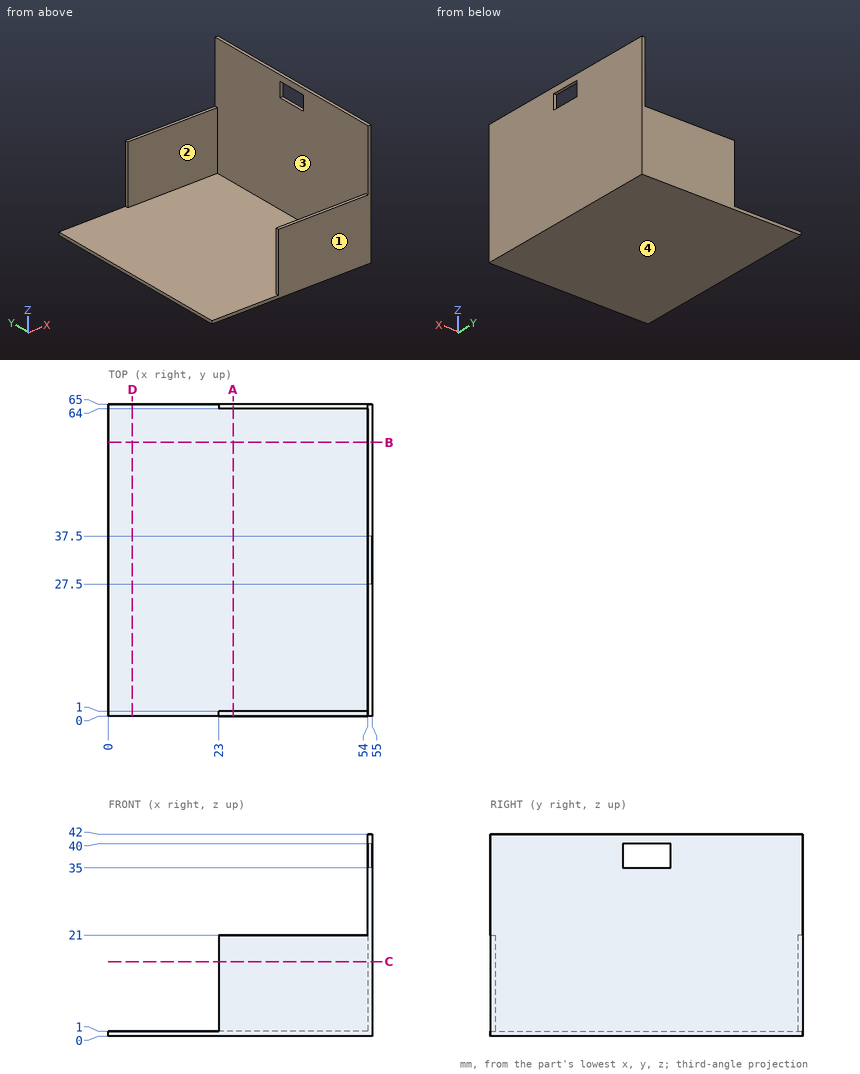
The drawing under review shows one solid part. Ordinate dimensions are in mm from its lowest x, y, z. Coordinates: 2 decimals unless noted, no trailing zeros. Write each loop counter-clockwise with the first axis right and the second up, starting at its lowest first coordinate (ties: lowest second). Pieces come first, ordered by that corner, then holes. Notation, with made-up numbers: (89, 38) -> (120, 38) arc R23 cw to (120, 47) -> close; hole circle Ø10 at (-24.75, 53). An arc over 180 degrees is marked (long way). One line per item, written item: value. Start each with the question number.
Q1. Clearance check with flat-ended pins moving along their axes: P1, Ø10, axis at x = 49.5, y = 6.5, coming from the +Z side; P2, Ø12, axis at y = 7.5, z = 32.5, coming from the -X side; P3, Ø10, axis at x = 20, y = 23.5, coming from the +Z side; P4, Ø0.8, axis at x = 45.5, y = 64.5, coming from the +Z side. State where each tip first meets the part, or that it passes through.
Q2. Add section B-B, the plane y = 57. Give the boundary of the cut face in (x, z), then the cut area to 3 significant figures.
Q3. To check wall thickness, follow probe 1 along Y at (x, z) = (30, 4.5); probe 2 along X at (y, z) = (61, 37.5); probe 3 along Z at (x, y) = (20, 58). State the ranges of each line that lie inside material, in increasing order.
Q4. Add section A-A, the plane x = 26. Give the boundary of the cut face in (y, z), then the cut area to 3 significant figures.
Q5. Add section C-C, the plane z = 15.5. Give the boundary of the cut face in (x, y), then the cut area to 3 significant figures.
Q6. Add section D-D, the plane x = 5. Give the boundary of the cut face in (y, z), then the cut area to 3 significant figures.
Q7. The part is to be moulded in two halves that separate along Y. For the marked faces 1, 2, 3 and 4, say which applies: +Y half, -Y half, draft (parallel to the pull), parting line (faces both ways), or undercut.
Response:
1. P1: z = 42
1. P2: x = 54
1. P3: z = 1
1. P4: z = 21
2. outline: (0, 0) -> (55, 0) -> (55, 42) -> (54, 42) -> (54, 1) -> (0, 1) -> close
2. area: 96.0 mm²
3. probe 1: 0 to 1, 64 to 65
3. probe 2: 54 to 55
3. probe 3: 0 to 1
4. outline: (0, 0) -> (65, 0) -> (65, 21) -> (64, 21) -> (64, 1) -> (1, 1) -> (1, 21) -> (0, 21) -> close
4. area: 105 mm²
5. outline: (23, 0) -> (55, 0) -> (55, 65) -> (23, 65) -> (23, 64) -> (54, 64) -> (54, 1) -> (23, 1) -> close
5. area: 127 mm²
6. outline: (0, 0) -> (65, 0) -> (65, 1) -> (0, 1) -> close
6. area: 65.0 mm²
7. face 1: -Y half
7. face 2: undercut
7. face 3: undercut
7. face 4: draft
